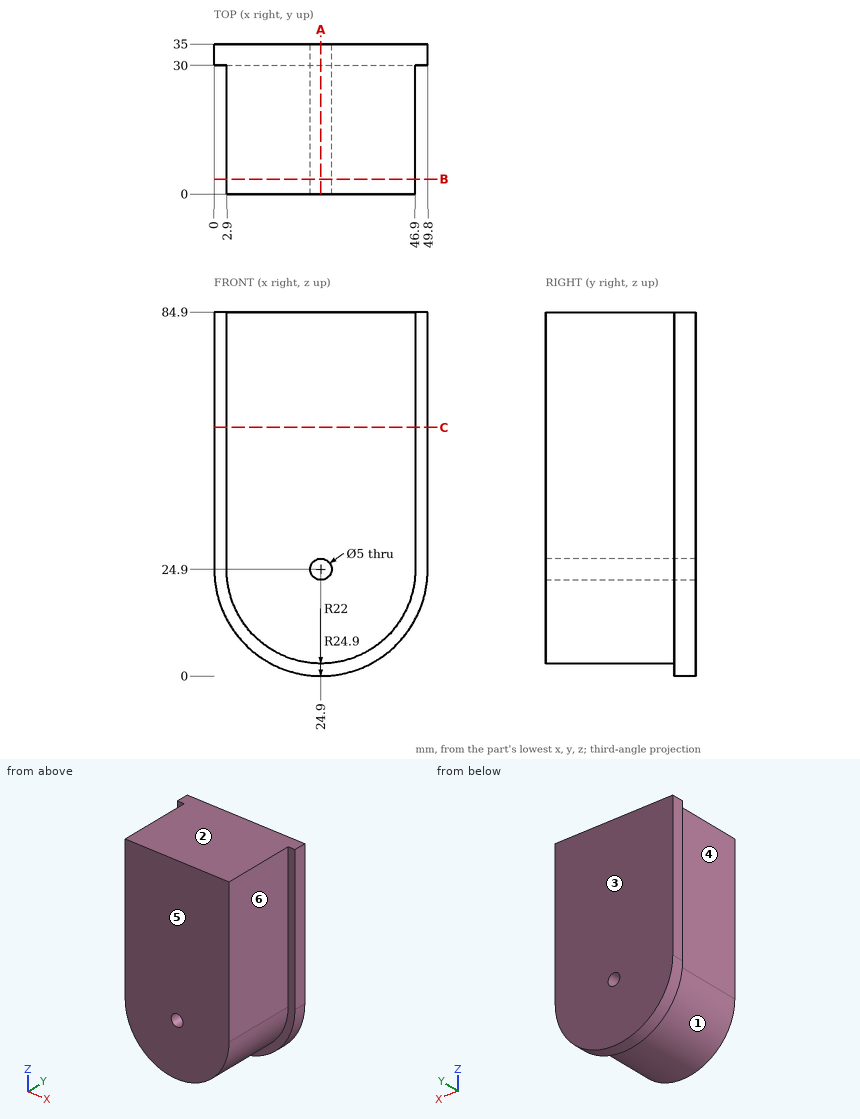
Geometry: see drawing. Coordinates: mm, zero at the bounding-box minimum. A direction names the side the tool comes from. Round coordinates to 2 decimals unless told otherwise and drop trailing zeros. Write each loop counter-clockwise with the first axis right and the second up, starting at its lowest first coordinate (ties: lowest second). Pieces come first, ordered by that corner, then holes.
1) Cut plane B-B (y = 3.5). Return the cut outline in (x, z), then the cut area to 3 significant figures.
2) Cut plane A-A (x = 24.9). Return the cut outline in (y, z).
3) Cut plane C-C (z = 58). Return the cut outline in (x, y), then the cut area to 3 significant figures.
4) Reachability of the marked faces 4, 5 and 6 from +Z, -Z, +X, -X, +Y, -Y: full face, straight path, thin tool, end or side. Return the list, or none.
5) Contact query for flat-ended pins moving along their axis: P1, Ø5, axis at y = 27, z = 36, coming from the -X side; P2, Ø3, axis at y = 31.5, z = 22, coming from the +X side; P3, Ø1.5, axis at x = 33, y = 23.5, coming from the -Z side. Output: stop coordinate, or through.
6) Draft query along Z for the marked faces 1, 2 and 3. Return one class per face: pulls with the +Z half, pulls with the -Z half, needs draft (parallel to the pull), parting line crosses it, or undercut.
7) Ray query, L1, parallel to X at y = 17, z = 51.5; L2, parallel to Z at x = 24, y = 20; L3, parallel to Z at x = 26, y = 30.5 (3 decimals). Return the intervals inside material, ascending.
Geometry says:
1. outline: (2.9, 24.9) arc R22 ccw to (46.9, 24.9) - (46.9, 84.9) - (2.9, 84.9) - close; hole circle Ø5 at (24.9, 24.9)
1. area: 3,380 mm2
2. outline: (0, 2.9) - (30, 2.9) - (30, 0) - (35, 0) - (35, 22.4) - (0, 22.4) - close; (0, 27.4) - (35, 27.4) - (35, 84.9) - (0, 84.9) - close
3. outline: (0, 30) - (2.9, 30) - (2.9, 0) - (46.9, 0) - (46.9, 30) - (49.8, 30) - (49.8, 35) - (0, 35) - close
3. area: 1,570 mm2
4. face 4: +Z, -Z, -X, -Y
4. face 5: +Z, -Z, +X, -X, -Y
4. face 6: +Z, -Z, +X, -Y
5. P1: stops at x = 2.9
5. P2: stops at x = 49.76
5. P3: stops at z = 4.16
6. face 1: pulls with the -Z half
6. face 2: pulls with the +Z half
6. face 3: needs draft
7. L1: x = 2.9 to 46.9
7. L2: z = 2.92 to 22.57, 27.23 to 84.9
7. L3: z = 0.024 to 22.655, 27.145 to 84.9
